```python
from build123d import *

# Parameters (mm, degrees)
PROFILES_R    = 10.25
PROFILES_R_2  = 6
PROFILE_DEPTH = 1
OUTERC_SIZE   = 0.1
INNERC_SIZE   = 0.1


with BuildPart() as part:
    # ProfileS → Profile (new body)
    with BuildSketch(Plane(origin=(0, 0, 0), x_dir=(1, 0, 0), z_dir=(0, 1, 0))):
        with Locations(Location((0, 0, 0), (0, 0, 270))):
            Circle(PROFILES_R)
        with Locations(Location((0, 0, 0), (0, 0, 270))):
            Circle(PROFILES_R_2, mode=Mode.SUBTRACT)
    extrude(amount=PROFILE_DEPTH)

    # OuterC
    outerc_edges = [part.edges().sort_by_distance(p)[0] for p in [
        (0, 0, -10.25),
        (0, 1, -10.25),
    ]]
    chamfer(outerc_edges, length=OUTERC_SIZE)

    # InnerC
    innerc_edges = [part.edges().sort_by_distance(p)[0] for p in [
        (0, 0, -6),
        (0, 1, -6),
    ]]
    chamfer(innerc_edges, length=INNERC_SIZE)


solid = part.part
```
Geometry: final body of the model. Coordinates: model frame, mm. Coordinates: 2 decimals unless noted, no trailing zeros. Order: outer loops, then holes, each group sorted by start corner. A loop starts at its lowest first (then second) coordinate and runs counter-clockwise, first axis right, second up. Notation, with made-up numbers: (1.25, 50) -> (44.25, 50) arc R22 cw to (44.25, 80) -> close; hole circle Ø10 at (-24.75, 10). An arc over 180 degrees is marked (long way). Write each question's results on one line, items separated by ' | '. Start each with the question number.
1) Cut plane B-B, the plane x = 0. Output: boundary loops of the cut face in (y, z), and give its area (3 significant figures).
2) Cut plane C-C, the plane y = 0.6. Output: boundary loops of the cut face in (x, z).
3) Material intervals for line 1 along X through (y, z) = (0.4, 0); line 2 along Z through (x, y) = (3, 0.5); line 3 along Z through (x, y) = (1, 0.65), sorted ascending.
4) Mould query, pull axis Z, two halves, no side actions, for faces 1 (the cylindrical face through (1.802, 0.494, 5.723)), 2 (the cylindrical face through (-10.006, 0.494, -2.222)), 3 (the flat face through (-7, 1, 0)). Classes: released by +Z, released by -Z, zero draft, split by the parting line, or undercut.
5) Cut plane A-A, the plane z = 0. Output: boundary loops of the cut face in (x, y).
Checks:
1) outline: (0, -10.15) -> (0.1, -10.25) -> (0.9, -10.25) -> (1, -10.15) -> (1, -6.1) -> (0.9, -6) -> (0.1, -6) -> (0, -6.1) -> close; (0, 6.1) -> (0.1, 6) -> (0.9, 6) -> (1, 6.1) -> (1, 10.15) -> (0.9, 10.25) -> (0.1, 10.25) -> (0, 10.15) -> close | area: 8.46 mm^2
2) outline: circle Ø20.5 at (0, 0); hole circle Ø12 at (0, 0)
3) line 1: -10.25 to -6, 6 to 10.25 | line 2: -9.8 to -5.2, 5.2 to 9.8 | line 3: -10.2 to -5.92, 5.92 to 10.2
4) face 1: undercut | face 2: split by the parting line | face 3: zero draft
5) outline: (-10.25, 0.1) -> (-10.15, 0) -> (-6.1, 0) -> (-6, 0.1) -> (-6, 0.9) -> (-6.1, 1) -> (-10.15, 1) -> (-10.25, 0.9) -> close; (6, 0.1) -> (6.1, 0) -> (10.15, 0) -> (10.25, 0.1) -> (10.25, 0.9) -> (10.15, 1) -> (6.1, 1) -> (6, 0.9) -> close
